The model under review builds one solid part; all positions refer to its coordinate system, in mm. A direction names the side the tool comes from. Give positions to 0.01 mm unless a question says otherwise; leave off trailing zeros. Loops run counter-clockwise (first coordinate to the right, second up) from the corner with the lowest first, then second, coordinate; pieces in that order, holes last. Notation, with made-up numbers: M 83,41.5 L 139,41.5 A22 ccw 139,48.5 Z; hole C 25,25 d11. An arc over 180 degrees is marked long. Write item = value, one per line. Start each with the question number.
1. For faces 4 (the face through (115.95, 17.54, 11.47)), 5 (the face through (20, 10, 12)), 6 (the face through (61, 33, 24.5)), 7 (the face through (115, 0, 12)), 8 (the face through (102, 30, 12)), list the 3-axis set-ups (+Z, -Z, +X, -X, +Y, -Y) from which the entire face can be reached by the end or side of a thin tool; tool diameter is ignored.
2. Wall thickness on line 1 along X through (y, z) = (17.85, 12.25); line 2 along X through (y, z) = (37, 12.25); line 3 along Y through (x, z) = (31, 12): over which ranges is each line inside the solid? List them lowest first. Write a range as from..to.
3. We need section A-A on y = 18.5. Give the boundary of the cut face in (x, z).
4. We need section C-C on x = 45.5. Give the boundary of the cut face in (y, z), then the cut area to 3 significant figures.
5. We need section B-B on z = 12.25. Count the separate pieces of the cut face and the enclosed holes in it, then the cut area to 3 significant figures.
6. Draft analysis for pull direction X (two halves, no side actions). For faces 1 (the face through (109, 28, 21.5)), 2 (the face through (97.294, 26.434, 12.408)), 3 (the face through (120, 10, 12)), state which applies: pulls with the +X half, pulls with the -X half, needs draft (parallel to the pull), parting line crosses it, or undercut.
7. For pin 1 (9.5 mm diameter, centred on x = 11, z = 15, fed in from +Y); pin 2 (5 mm diameter, centred on x = 10, z = 12.25, fed in from +Y); pin 3 (9 mm diameter, centred on y = 34, z = 8, fed in from +X); pin 4 (10.5 mm diameter, centred on x = 110, z = 12.25, fed in from -Y), all flat-tipped, find the tip position at first contact; note any pin that passes through.
from build123d import *

# Parameters (mm, degrees)
EXTRUDE_1_DEPTH     = 24.5
FILLET_1_R          = 20
FILLET_2_R          = 9
SKETCH_2_W          = 18.5
SKETCH_2_H          = 26.060105981
CUT_EXTRUDE_1_DEPTH = 18
SKETCH_3_W          = 18.5
SKETCH_3_H          = 21.487076152
CUT_EXTRUDE_2_DEPTH = 18
FILLET_3_R          = 1
SKETCH_6_R          = 4
CUT_EXTRUDE_3_DEPTH = 129.841957452
SKETCH_7_R          = 6
CUT_EXTRUDE_4_DEPTH = 5


with BuildPart() as part:
    # Эскиз1 → Бобышка-Вытянуть1 (new body)
    with BuildSketch(Plane.XY):
        Polygon((0, 0), (0, 40), (120, 40), (120, 0), (100, 0), (100, 29), (20, 29), (20, 0), align=None)
    extrude(amount=EXTRUDE_1_DEPTH)

    # Скругление1
    fillet_1_edges = [part.edges().sort_by_distance(p)[0] for p in [
        (0, 40, 12.25),
        (120, 40, 12.25),
    ]]
    fillet(fillet_1_edges, radius=FILLET_1_R)

    # Скругление2
    fillet_2_edges = [part.edges().sort_by_distance(p)[0] for p in [
        (100, 29, 12.25),
        (20, 29, 12.25),
    ]]
    fillet(fillet_2_edges, radius=FILLET_2_R)

    # Эскиз2 → Вырез-Вытянуть1 (cut)
    with BuildSketch(Plane(origin=(120, 0, 0), x_dir=(0, 0, -1), z_dir=(1, 0, 0))):
        with Locations((-12.25, 33.03005299)):
            Rectangle(SKETCH_2_W, SKETCH_2_H)
    extrude(amount=-CUT_EXTRUDE_1_DEPTH, mode=Mode.SUBTRACT)

    # Эскиз3 → Вырез-Вытянуть2 (cut)
    with BuildSketch(Plane.ZY):
        with Locations((12.25, 30.743538076)):
            Rectangle(SKETCH_3_W, SKETCH_3_H)
    extrude(amount=-CUT_EXTRUDE_2_DEPTH, mode=Mode.SUBTRACT)

    # Скругление3
    fillet_3_edges = [part.edges().sort_by_distance(p)[0] for p in [
        (20, 10, 0),
        (120, 10, 24.5),
        (0, 10, 0),
        (0, 10, 24.5),
        (60, 40, 0),
        (114.142135624, 34.142135624, 0),
        (5.857864376, 34.142135624, 0),
        (60, 40, 24.5),
        (114.142135624, 34.142135624, 24.5),
        (5.857864376, 34.142135624, 24.5),
        (60, 29, 0),
        (60, 29, 24.5),
        (100, 10, 0),
        (100, 10, 24.5),
        (22.636038969, 26.363961031, 0),
        (22.636038969, 26.363961031, 24.5),
        (97.363961031, 26.363961031, 0),
        (97.363961031, 26.363961031, 24.5),
        (20, 10, 24.5),
        (120, 10, 0),
    ]]
    fillet(fillet_3_edges, radius=FILLET_3_R)

    # Эскиз6 → Вырез-Вытянуть3 (cut, through all)
    with BuildSketch(Plane(origin=(0, 0, 0), x_dir=(-1, 0, 0), z_dir=(0, -1, 0))):
        with Locations(Location((-10, -12.25, 0), (0, 0, 180))):
            Circle(SKETCH_6_R)
        with Locations(Location((-110, -12.25, 0), (0, 0, 180))):
            Circle(SKETCH_6_R)
    extrude(amount=-CUT_EXTRUDE_3_DEPTH, mode=Mode.SUBTRACT)

    # Эскиз7 → Вырез-Вытянуть4 (cut)
    with BuildSketch(Plane(origin=(0, 20, 0), x_dir=(1, 0, 0), z_dir=(0, 1, 0))):
        with Locations(Location((10, -12.25, 0), (0, 0, 270))):
            Circle(SKETCH_7_R)
        with Locations(Location((110, -12.25, 0), (0, 0, 270))):
            Circle(SKETCH_7_R)
    extrude(amount=-CUT_EXTRUDE_4_DEPTH, mode=Mode.SUBTRACT)


solid = part.part
Final values:
q1.face_4 = +Y
q1.face_5 = +Z, -Z, -Y
q1.face_6 = +Z, +X, -X, +Y, -Y
q1.face_7 = +Z, -Z, +X, -X, -Y
q1.face_8 = +X, +Y
q2.line_1 = 0..4, 16..20, 100..104, 116..120
q2.line_2 = 18..102
q2.line_3 = 29..40
q3.outline = M 0,1 A1 ccw 1,0 L 19,0 A1 ccw 20,1 L 20,23.5 A1 ccw 19,24.5 L 1,24.5 A1 ccw 0,23.5 Z; M 100,1 A1 ccw 101,0 L 119,0 A1 ccw 120,1 L 120,23.5 A1 ccw 119,24.5 L 101,24.5 A1 ccw 100,23.5 Z; hole C 10,12.25 d12; hole C 110,12.25 d12
q4.outline = M 29,1 A1 ccw 30,0 L 39,0 A1 ccw 40,1 L 40,23.5 A1 ccw 39,24.5 L 30,24.5 A1 ccw 29,23.5 Z
q4.area = 269 mm²
q5.separate_pieces = 3
q5.enclosed_holes = 0
q5.area = 1,430 mm²
q6.face_1 = needs draft
q6.face_2 = undercut
q6.face_3 = pulls with the +X half
q7.pin_1 = 20
q7.pin_2 = through
q7.pin_3 = 102
q7.pin_4 = 0
